Autodesk Inventor part; units mm, degrees
ref_plane "YZ Plane" through (0, 0, 0) normal (1, 0, 0) x (0, 1, 0)
ref_plane "XZ Plane" through (0, 0, 0) normal (0, 1, 0) x (-1, 0, 0)
ref_plane "XY Plane" through (0, 0, 0) normal (0, 0, 1) x (1, 0, 0)
sketch "Boceto1" plane through (0, 0, 0) normal (0, 0, 1) x (1, 0, 0)
  line L0 (0, 0) -> (8, 0)
  line L1 (30, 0) -> (37, 0)
  arc A0 (30, 0) -> (8, 0) centre (19, 0) ccw
  line L2 (0, 0) -> (0, 8)
  line L3 (0, 8) -> (6.3114, 8)
  line L4 (37, 0) -> (37, 8)
  line L5 (37, 8) -> (31.6886, 8)
  arc A1 (31.6886, 8) -> (6.3114, 8) centre (19, 0) ccw
  line L6 (19, 11) -> (19, 15) construction
  dimension "d0" = 11
  dimension "d1" = 37
  dimension "d2" = 8
  dimension "d3" = 8
  dimension "d5" = 4
extrude "Extrusión1" add sketch "Boceto1" along normal blind 10
sketch "Boceto3" plane through (0, 0, 0) normal (0, -1, 0) x (1, 0, 0)
  line L0 (0, 0) -> (8, 0)
  line L1 (0, 0) -> (0, 10)
  line L2 (30, 0) -> (30, 10)
  line L3 (30, 0) -> (37, 0)
  circle A0 centre (4, 5) radius 2.05
  circle A1 centre (33.5, 5) radius 2.05
  point P0 (0, 5)
  point P1 (30, 5)
  point P2 (4, 0)
  point P3 (33.5, 0)
  dimension "d12" = 4.1
  dimension "d13" = 4.1
extrude "Extrusión3" cut sketch "Boceto3" against normal through all
properties part number "SoporteMotorCierre"
Build history of the part. All positions in model axes, mm. A direction names the side the tool comes from. Give positions to 0.01 mm unless a question says otherwise; leave off trailing zeros. Loops run counter-clockwise (first coordinate to the right, second up) from the corner with the lowest first, then second, coordinate; pieces in that order, holes last.
Item 1: Flat gauge pins, fed straight in: pin 1 (3 mm diameter, centred on x = 25, z = 2.5, fed in from -Y); pin 2 (2.5 mm diameter, centred on x = 33.5, z = 3, fed in from +Y); pin 3 (1.5 mm diameter, centred on y = 9, z = 5, fed in from -X); pin 4 (8 mm diameter, centred on x = 23.5, y = 1.5, fed in from +Z). Where does each tip first touch, or does it go through?
Answers follow:
pin 1: stops at y = 8.05
pin 2: stops at y = 8
pin 3: stops at x = 6.47
pin 4: passes through
Item 2: Slice it at B-B, the plane y = 6.5. List the corners of the cut face in (x, z).
Answers follow:
outline: (0, 0) - (10.13, 0) - (10.13, 10) - (0, 10) - close; (27.87, 0) - (37, 0) - (37, 10) - (27.87, 10) - close; hole circle Ø4.1 at (4, 5); hole circle Ø4.1 at (33.5, 5)
Item 3: Pull direction Z, two halves, no side cores. Call faces 1 (the face through (22, 11, 0)), 2 (the face through (19, 11, 5)), 3 (the face through (31.45, 4.12, 5.09)): released by +Z, released by -Z, zero draft, split by the parting line, or undercut.
Answers follow:
face 1: released by -Z
face 2: zero draft
face 3: undercut
Item 4: Which spindle directions (+Z, -Z, +X, -X, +Y, -Y) get a long thin tool onto all of the face, cutting with end or side? Do faces 4 (the face through (1.7, 8, 4.9)), 5 (the face through (36, 8, 5)), 6 (the face through (2, 0, 4)). Say none if no direction does.
Answers follow:
face 4: +Z, -Z, -X, +Y
face 5: +Z, -Z, +X, +Y
face 6: +Z, -Z, +X, -X, -Y
Item 5: Slice it at D-D, the plane y = 10. List the corners of the cut face in (x, z), and give its area (3 significant figures).
Answers follow:
outline: (7.82, 0) - (14.42, 0) - (14.42, 10) - (7.82, 10) - close; (23.58, 0) - (30.18, 0) - (30.18, 10) - (23.58, 10) - close
area: 132 mm2
Item 6: Slice it at C-C, the plane z = 2.25. List the corners of the cut face in (x, y), and give its area (3 significant figures).
Answers follow:
outline: (0, 0) - (8, 0) arc R11 cw to (30, 0) - (37, 0) - (37, 8) - (31.69, 8) arc R15 ccw to (6.31, 8) - (0, 8) - close
area: 231 mm2
Item 7: Drill centre lines: line 1 (Z direction, x = 33.5, y = 3.75); line 2 (X direction, y = 5.5, z = 6.75); line 3 (Y direction, x = 35.5, z = 2.5). Where is each one in solid material? Low to high.
Answers follow:
line 1: z = 0 to 2.95, 7.05 to 10
line 2: x = 0 to 2.93, 5.07 to 9.47, 28.53 to 32.43, 34.57 to 37
line 3: y = 0 to 8
Item 8: Slice it at A-A, the plane x = 33.5. List the corners of the cut face in (y, z).
Answers follow:
outline: (0, 0) - (8, 0) - (8, 2.95) - (0, 2.95) - close; (0, 7.05) - (8, 7.05) - (8, 10) - (0, 10) - close
